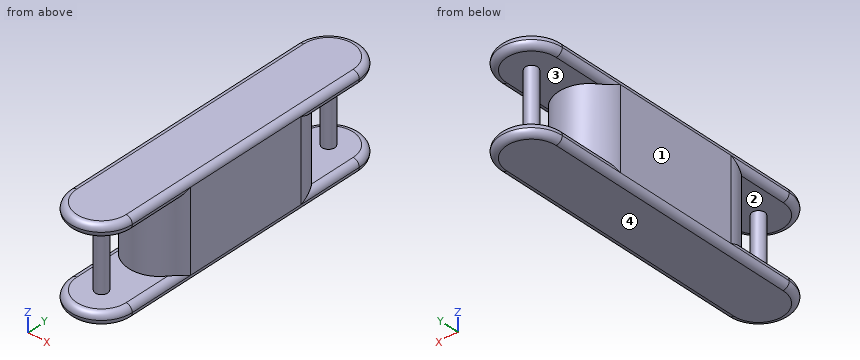
from build123d import *

# Parameters (mm, degrees)
SKETCH3_W           = 100
SKETCH3_H           = 300
BOSS_EXTRUDE1_DEPTH = 75
CUT_EXTRUDE1_REACH  = 422.463
CUT_EXTRUDE1_START  = -150
SKETCH4_W           = 100
SKETCH4_H           = 110
SKETCH6_R           = 10
BOSS_EXTRUDE2_DEPTH = 55
CUT_EXTRUDE2_REACH  = 422.463
CUT_EXTRUDE2_START  = 150
SKETCH4_2_W         = 100
SKETCH4_2_H         = 110
FILLET1_RADIUS      = 50
FILLET1_LENGTH      = 110
FILLET2_RADIUS      = 50
FILLET2_LENGTH      = 110
FILLET3_R           = 10


with BuildPart() as part:
    # Sketch3 → Boss-Extrude1 (new, symmetric)
    with BuildSketch(Plane.XY):
        Rectangle(SKETCH3_W, SKETCH3_H)
        with BuildLine():
            Line((-50, -150), (-50, -205))
            ThreePointArc((-50, -205), (0, -255), (50, -205))
            Line((50, -205), (50, -150))
            Line((50, -150), (-50, -150))
        make_face()
        with BuildLine():
            ThreePointArc((-50, 205), (0, 255), (50, 205))
            Line((50, 205), (50, 150))
            Line((50, 150), (-50, 150))
            Line((-50, 150), (-50, 205))
        make_face()
    extrude(amount=BOSS_EXTRUDE1_DEPTH, both=True)

    # Sketch4 → Cut-Extrude1 (cut, up to next)
    with BuildSketch(Plane(origin=(0, 0, 0), x_dir=(1, 0, 0), z_dir=(0, 1, 0)).offset(CUT_EXTRUDE1_START), mode=Mode.PRIVATE) as cut_extrude1_sk1:
        Rectangle(SKETCH4_W, SKETCH4_H)
    cut_extrude1_tool1 = extrude(cut_extrude1_sk1.sketch, amount=-CUT_EXTRUDE1_REACH, mode=Mode.PRIVATE) & part.part
    add(cut_extrude1_tool1.solids().sort_by_distance((0, -150, 0))[0], mode=Mode.SUBTRACT)

    # Sketch6 → Boss-Extrude2 (add, symmetric)
    with BuildSketch(Plane.XY):
        with Locations(Location((0, -205, 0), (0, 0, 180))):
            Circle(SKETCH6_R)
    boss_extrude2 = extrude(amount=BOSS_EXTRUDE2_DEPTH, both=True)

    # Sketch4<2> → Cut-Extrude2 (cut, up to next)
    with BuildSketch(Plane(origin=(0, 0, 0), x_dir=(1, 0, 0), z_dir=(0, 1, 0)).offset(CUT_EXTRUDE2_START), mode=Mode.PRIVATE) as cut_extrude2_sk1:
        Rectangle(SKETCH4_2_W, SKETCH4_2_H)
    cut_extrude2_tool1 = extrude(cut_extrude2_sk1.sketch, amount=CUT_EXTRUDE2_REACH, mode=Mode.PRIVATE) & part.part
    add(cut_extrude2_tool1.solids().sort_by_distance((0, 150, 0))[0], mode=Mode.SUBTRACT)

    # Mirror2: Boss-Extrude2 across plane
    add(boss_extrude2.mirror(Plane.ZX))

    # Fillet1: full round fillet: the end face becomes a half cylinder, R = half its width
    fillet1_face = Plane((0, 150, 0), x_dir=(0, 0, -1), z_dir=(0, 1, 0))  # on the end face: x along it, z out of the body
    fillet1_slab = fillet1_face.offset(-FILLET1_RADIUS / 2) * Box(FILLET1_LENGTH, 2 * FILLET1_RADIUS, FILLET1_RADIUS, mode=Mode.PRIVATE)  # the body's end, R deep
    fillet1_round = Plane((0, 100, 0), x_dir=(0, 1, 0), z_dir=(0, 0, -1)) * Cylinder(FILLET1_RADIUS, FILLET1_LENGTH, mode=Mode.PRIVATE)  # its axis R under the face
    add(fillet1_slab - fillet1_round, mode=Mode.SUBTRACT)

    # Fillet2: full round fillet: the end face becomes a half cylinder, R = half its width
    fillet2_face = Plane((0, -150, 0), x_dir=(0, 0, 1), z_dir=(0, -1, 0))  # on the end face: x along it, z out of the body
    fillet2_slab = fillet2_face.offset(-FILLET2_RADIUS / 2) * Box(FILLET2_LENGTH, 2 * FILLET2_RADIUS, FILLET2_RADIUS, mode=Mode.PRIVATE)  # the body's end, R deep
    fillet2_round = Plane((0, -100, 0), x_dir=(0, -1, 0), z_dir=(0, 0, 1)) * Cylinder(FILLET2_RADIUS, FILLET2_LENGTH, mode=Mode.PRIVATE)  # its axis R under the face
    add(fillet2_slab - fillet2_round, mode=Mode.SUBTRACT)

    # Fillet3
    fillet3_edges = [part.edges().sort_by_distance(p)[0] for p in [
        (-50, -152.5, 55),
        (0, -255, 55),
        (-50, -152.5, -55),
        (0, -255, -55),
        (-50, 152.5, 55),
        (0, 255, 55),
        (-50, 152.5, -55),
        (0, 255, -55),
        (0, 255, -75),
        (-50, 0, -75),
        (0, -255, -75),
        (50, 0, -75),
        (0, 255, 75),
        (50, 0, 75),
        (0, -255, 75),
        (-50, 0, 75),
        (50, -152.5, 55),
        (50, -152.5, -55),
        (50, 152.5, 55),
        (50, 152.5, -55),
    ]]
    fillet(fillet3_edges, radius=FILLET3_R - 0.0001)  # a hair under: the kernel refuses the full size


solid = part.part
Model file for the job. Use its own axes, mm. Face numbers are marked on the shaded views. A direction names the side the tool comes from. Coordinates: 2 decimals unless noted, no trailing zeros. Loops run counter-clockwise (first coordinate to the right, second up) from the corner with the lowest first, then second, coordinate; pieces in that order, holes last. Notation, with made-up numbers: (53.5, -16.5) -> (100.5, -16.5) arc R24 cw to (100.5, 2.5) -> close; hole circle Ø10 at (35, 78). An arc over 180 degrees is marked (long way). Use one line per item in the form item = value. Start each with the question number.
(1) Tool access for the marked faces 1 and 2: list every direction of +Z, -Z, +X, -X, +Y, -Y with a clear straight run to the whole face (end or side of a thin tool).
(2) Probe probe 1 along Z at (x, y) = (-31, 177); probe 2 along Z at (x, y) = (-42, 134.5); probe 3 along X at (y, z) = (102, 24.5). List the from-to ranges inside material, lowest first. Write a range as from..to.
(3) Flat gauge pins, fed straight in: pin 1 (6 mm diameter, centred on y = 131, z = -40, fed in from -X); pin 2 (4 mm diameter, centred on x = -38.5, z = 6.5, fed in from +Y); pin 3 (3 mm diameter, centred on x = 19, z = 58, fed in from -Y). Where does each tip first touch, or does it go through?
(4) Pull direction Y, two halves, no side cores. Call the marked faces 3 and 4: pulls with the +Y half, pulls with the -Y half, needs draft (parallel to the pull), parting line crosses it, or undercut.
(5) Cut at C-C on z = 28.5. Give the cut face in (x, y).
(6) Cut at B-B on x = 0. Give the number of separate pieces and of enclosed holes in the cut face, and give its area (3 significant figures).
Values:
q1.face_1 = +Z, -Z, -X, +Y, -Y
q1.face_2 = none
q2.probe_1 = -75..-55, 55..75
q2.probe_2 = -74.8..-55.2, 55.2..74.8
q2.probe_3 = -49.96..49.96
q3.pin_1 = -41.42
q3.pin_2 = 134.17
q3.pin_3 = -249.63
q4.face_3 = undercut
q4.face_4 = needs draft
q5.outline = (-50, -100) arc R50 ccw to (50, -100) -> (50, 100) arc R50 ccw to (-50, 100) -> close; circle Ø20 at (0, -205); circle Ø20 at (0, 205)
q6.separate_pieces = 1
q6.enclosed_holes = 2
q6.area = 57,600 mm2
